Check sheet for the modelled part. Datum: model origin and axes. Units: mm. Face numbers are marked on the shaded views. A direction names the side the tool comes from. Round coordinates to 2 decimals unless told otherwise and drop trailing zeros. Order: outer loops, then holes, each group sorted by start corner. A loop starts at its lowest first (then second) coordinate and runs counter-clockwise, first axis right, second up.
Q1. Depth check by flat-ended pin: P1, Ø3.5, axis at x = 7.5, y = 0, coming from the +Z side; P2, Ø1.1, axis at x = -6.5, y = 4, coming from the +Z side; P3, Ø2, axis at y = 4.5, z = 3.5, coming from the -X side. Enter the tip coordinate at first touch or a pass-through.
Q2. Scan lines: probe 1 along Y at (x, z) = (0, 1.05); probe 2 along Z at (x, y) = (0, 5.65); probe 3 along Z at (x, y) = (-7.25, 1.5). Record each from-to range of solid material in increasing order.
Q3. Cross-section at D-D on x = 3.5. Record the cut outline in (y, z).
Q4. Cross-section at C-C on y = -4.5. Record the cut outline in (x, z).
Q5. Cross-section at B-B on z = 0.8. Record the cut outline in (x, y), then the cut area to 3 significant figures.
Q6. Mould release check, pull along X, two halves, no side actions. Record for the marked faces 1, 2 and 3: +X half, -X half, draft (parallel to the pull), parting line (faces both ways), or undercut.
Q7. Set-up check for the marked faces 4 and 5: record each of +Z, -Z, +X, -X, +Y, -Y from which the full face is reachable in a straight line by a thin tool's end or side.
Q8. Cross-section at A-A on x = 0. Record the cut outline in (y, z).
Autodesk Inventor part; units mm, degrees
ref_plane "Work Plane3" through (0, 6, 0) normal (0, 1, 0) x (-1, 0, 0)
ref_plane "YZ Plane" through (0, 0, 0) normal (1, 0, 0) x (0, 1, 0)
ref_plane "XY Plane" through (0, 0, 0) normal (0, 0, 1) x (1, 0, 0)
sketch "Sketch2" plane through (0, 0, 0) normal (0, 0, 1) x (1, 0, 0)
  circle A0 centre (0, 0) radius 5.05
  circle A1 centre (-7.75, 0) radius 1.65
  circle A2 centre (-7.75, 0) radius 2.5
  circle A3 centre (0, 0) radius 6
  line L0 (-2.7097, 5.3533) -> (-8.879, 2.2305)
  line L1 (-8.879, -2.2305) -> (-2.7097, -5.3533)
  circle A4 centre (7.75, 0) radius 1.65
  circle A5 centre (7.75, 0) radius 2.5
  line L2 (2.7097, 5.3533) -> (8.879, 2.2305)
  line L3 (2.7097, -5.3533) -> (8.879, -2.2305)
  line L4 (0, 0) -> (7.75, 0) construction
  line L5 (0, 0) -> (-7.75, 0) construction
  dimension "d0" = 10.1
  dimension "d1" = 3.3
  dimension "d2" = 5
  dimension "d3" = 12
  dimension "d27" = 7.75
sketch "Sketch5" plane through (0, 0, 0) normal (0, 0, 1) x (1, 0, 0)
  circle A0 centre (0, 0) radius 6
  circle A1 centre (0, 0) radius 5.05
extrude "Extrusion5" add sketch "Sketch5" along normal blind 5
extrude "Extrusion6" add sketch "Sketch2" along normal blind 2 contours A0 | A2 A3 | L0 A3 A2 | A2 A3 L1 | A3 A5 A2 | A2 A3 | L2 A5 A3 | A3 A5 L3 | A5 A3 | A3 A5
sketch "Sketch6" plane through (0, 0, 2) normal (0, 0, 1) x (1, 0, 0)
  circle A0 centre (0, 0) radius 5.05
extrude "Extrusion7" cut sketch "Sketch6" against normal through all
sketch "Sketch7" plane through (0, 0, 2) normal (0, 0, 1) x (1, 0, 0)
  circle A0 centre (-7.75, 0) radius 1.65
  circle A1 centre (7.75, 0) radius 1.65
  point P0 (0, 0)
extrude "Extrusion9" add sketch "Sketch7" against normal blind 0.5
ref_plane "Work Plane3" through (0, 6, 0) normal (0, 1, 0) x (-1, 0, 0)
sketch "Sketch8" plane through (0, 6, 0) normal (0, 1, 0) x (-1, 0, 0)
  line L0 (-5.05, 0) -> (-5.05, 5)
  circle A0 centre (0, 2.5) radius 1.25
  point P0 (0, 0)
  point P1 (-5.05, 2.5)
  dimension "d24" = 2.5
extrude "Extrusion10" cut sketch "Sketch8" against normal blind 3
properties part number "ShaftCollarMagnetMount" material "ABS Plastic"
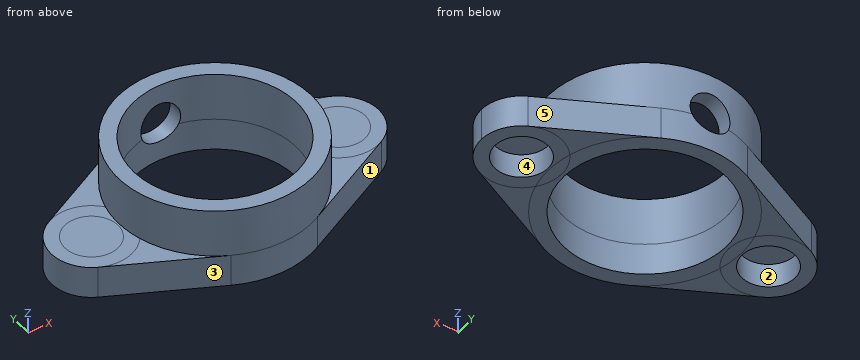
Results found:
1. P1: stops at z = 5
1. P2: stops at z = 2
1. P3: stops at x = -4.87
2. probe 1: y = -6 to -5.05, 5.05 to 6
2. probe 2: z = 0 to 1.25, 3.75 to 5
2. probe 3: z = 1.5 to 2
3. outline: (-4.95, 0) - (-3.64, 0) - (-3.64, 5) - (-4.87, 5) - (-4.87, 2) - (-4.95, 2) - close; (3.64, 0) - (4.95, 0) - (4.95, 2) - (4.87, 2) - (4.87, 5) - (3.64, 5) - close
4. outline: (-4.4, 0) - (-2.29, 0) - (-2.29, 5) - (-3.97, 5) - (-3.97, 2) - (-4.4, 2) - close; (2.29, 0) - (4.4, 0) - (4.4, 2) - (3.97, 2) - (3.97, 5) - (2.29, 5) - close
5. outline: (-8.88, -2.23) - (-2.71, -5.35) arc R6 ccw to (2.71, -5.35) - (8.88, -2.23) arc R2.5 ccw to (8.88, 2.23) - (2.71, 5.35) arc R6 ccw to (-2.71, 5.35) - (-8.88, 2.23) arc R2.5 ccw to start; hole circle Ø3.3 at (-7.75, 0); hole circle Ø10.1 at (0, 0); hole circle Ø3.3 at (7.75, 0)
5. area: 67.8 mm2
6. face 1: +X half
6. face 2: undercut
6. face 3: -X half
7. face 4: -Z
7. face 5: +Z, -Z, +X, +Y
8. outline: (-6, 0) - (-5.05, 0) - (-5.05, 5) - (-6, 5) - close; (5.05, 0) - (6, 0) - (6, 1.25) - (5.05, 1.25) - close; (5.05, 3.75) - (6, 3.75) - (6, 5) - (5.05, 5) - close
